```python
from build123d import *

# Parameters (mm, degrees)
F1_DEPTH    = 48
F2_DEPTH    = 10
F3_R        = 6
F4_T1_DEPTH = 30
F5_R        = 6
F6_DEPTH    = 3
F5_W        = 28
F5_H        = 5
F7_DEPTH    = 5
F8_DEPTH    = 25


# Not quite as in the source:
# - a fillet or chamfer that OpenCascade refuses, or shapes differently, is made with other operations: its cross-section is extruded or revolved along the edge and cut away or added


with BuildPart() as f1:
    # F0 (on Front) → F1 (new body)
    with BuildSketch(Plane.XZ):
        Polygon((-21, 43), (-31, 43), (-31, 13), (31, 13), (31, 43), (21, 43), (21, 23), (-21, 23), align=None)
    extrude(amount=F1_DEPTH)

    # F0 (on Front) → F2 (join)
    with BuildSketch(Plane.XZ):
        Polygon((-31, 43), (-46, 43), (-46, 0), (46, 0), (46, 43), (31, 43), (31, 13), (-31, 13), align=None)
        Polygon((-21, 43), (-31, 43), (-31, 13), (31, 13), (31, 43), (21, 43), (21, 23), (-21, 23), align=None)
    extrude(amount=F2_DEPTH)

    # F3
    f3_edges = [f1.edges().sort_by_distance(p)[0] for p in [
        (-46, -5, 0),
        (46, -5, 0),
    ]]
    fillet(f3_edges, radius=F3_R)

    # F4: fillet of radius 25 on 2 edges, made by hand

    # F4_s2 → F4_t1 (join)
    with BuildSketch(Plane.XY.offset(13)):
        with BuildLine():
            ThreePointArc((-46, -10), (-35.0834993366, -19.2198145372), (-31, -32.9128784748))
            Line((-31, -32.9128784748), (-31, -10))
            Line((-31, -10), (-46, -10))
        make_face()
        with BuildLine():
            ThreePointArc((46, -10), (35.0834993366, -19.2198145372), (31, -32.9128784748))
            Line((31, -32.9128784748), (31, -10))
            Line((31, -10), (46, -10))
        make_face()
    extrude(amount=F4_T1_DEPTH)

    # F5 (on face) → F6 (join)
    with BuildSketch(Plane(origin=(0, 0, 13), x_dir=(1, 0, 0), z_dir=(0, 0, -1))):
        with BuildLine():
            Line((14, 15), (14, 29))
            ThreePointArc((14, 29), (0, 43), (-14, 29))
            Line((-14, 29), (-14, 15))
            Line((-14, 15), (14, 15))
        make_face()
        with Locations((0, 29)):
            Circle(F5_R, mode=Mode.SUBTRACT)
    extrude(amount=F6_DEPTH)

    # F5 (on face) → F7 (join)
    with BuildSketch(Plane(origin=(0, 0, 13), x_dir=(1, 0, 0), z_dir=(0, 0, -1))):
        with Locations((0, 12.5)):
            Rectangle(F5_W, F5_H)
    extrude(amount=F7_DEPTH)

    # F5 (on face) → F8 (cut)
    with BuildSketch(Plane(origin=(0, 0, 13), x_dir=(1, 0, 0), z_dir=(0, 0, -1))):
        with Locations((0, 29)):
            Circle(F5_R)
    extrude(amount=-F8_DEPTH, mode=Mode.SUBTRACT)


solid = f1.part
```
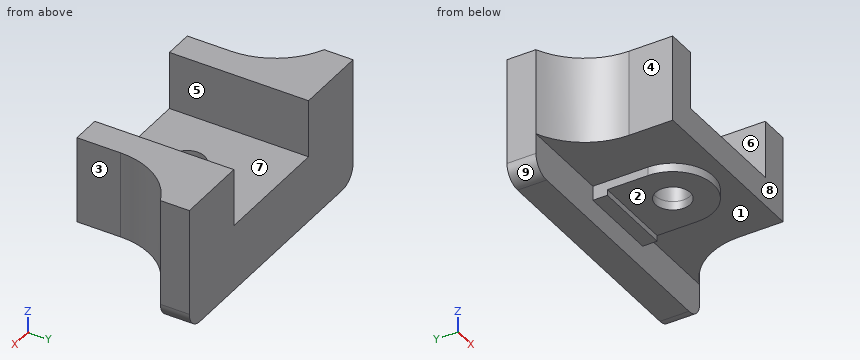
Work out the finished part from the listing and answer in its coordinate system (mm). Face numbers are marked on the shaded views. A direction names the side the tool comes from. Give positions to 0.01 mm unless a question says otherwise; leave off trailing zeros. Loops run counter-clockwise (first coordinate to the right, second up) from the corner with the lowest first, then second, coordinate; pieces in that order, holes last. Notation, with made-up numbers: (16.25, 37) -> (24.25, 37) arc R10 cw to (24.25, 43) -> close; hole circle Ø3 at (-37.75, 19.5). An arc over 180 degrees is marked (long way). Put each result on its own line as item: value. Start each with the question number.
Item 1: The part is cut by section B-B (z = 14). Give the vertices of the cut face in (x, y).
Item 2: Each of these flat-tipped pins is pushed along its axis until it touches: P1, Ø7.5, axis at y = -37.5, z = 29.5, coming from the -X side; P2, Ø4, axis at x = 4.5, y = -13, coming from the -Z side; P3, Ø12, axis at y = -33, z = 29.5, coming from the -X side. Where does it stop, or does it pass through?
Item 3: The part is cut by section D-D (y = -38). Give the vertices of the cut face in (x, z), then the cut area to 3 significant figures.
Item 4: Find the intervals of material crossed by L1, parallel to Y at x = 0, z = 20; L2, parallel to Y at x = 0, z = 10.95; L3, parallel to X at y = -3.5, z = 25, in increasing order. Write a range as [from, to].
Item 5: The mould has two halves that part along X. Classify the marked faces 6, 7, 8 and 9: released by +X, released by -X, zero draft, split by the parting line, or undercut.
Item 6: The part is cut by section C-C (y = -26). Give the vertices of the cut face in (x, z), then the cut area to 3 significant figures.
Item 7: Which of the six approach directions +Z, -Z, +X, -X, +Y, -Y give full straight-line access (tool end or side, diameter ignored) to the marked faces 1, 2, 3, 4 and 5?
Item 8: The part is cut by section A-A (x = 0). Give the vertices of the cut face in (y, z).
Answers below:
1. outline: (-46, -10) arc R25 cw to (-31, -32.91) -> (-31, -48) -> (31, -48) -> (31, -32.91) arc R25 cw to (46, -10) -> (46, 0) -> (-46, 0) -> close; hole circle Ø12 at (0, -29)
2. P1: x = -31
2. P2: z = 8
2. P3: x = -31.71
3. outline: (-31, 13) -> (-10.72, 13) -> (-10.72, 10) -> (10.72, 10) -> (10.72, 13) -> (31, 13) -> (31, 43) -> (21, 43) -> (21, 23) -> (-21, 23) -> (-21, 43) -> (-31, 43) -> close
3. area: 1,080 mm2
4. L1: [-48, -35], [-23, 0]
4. L2: [-43, -35], [-23, 0]
4. L3: [-46, -21], [21, 46]
5. face 6: undercut
5. face 7: undercut
5. face 8: zero draft
5. face 9: released by -X
6. outline: (-31.97, 13) -> (-14, 13) -> (-14, 10) -> (-5.2, 10) -> (-5.2, 23) -> (-21, 23) -> (-21, 43) -> (-31.97, 43) -> close; (5.2, 10) -> (14, 10) -> (14, 13) -> (31.97, 13) -> (31.97, 43) -> (21, 43) -> (21, 23) -> (5.2, 23) -> close
6. area: 1,030 mm2
7. face 1: -Z, -Y
7. face 2: -Z, +X, -X, -Y
7. face 3: +Z, -Z, +X, -Y
7. face 4: +Z, -Z, -X, -Y
7. face 5: +Z, +Y, -Y
8. outline: (-48, 13) -> (-43, 13) -> (-43, 10) -> (-35, 10) -> (-35, 23) -> (-48, 23) -> close; (-23, 10) -> (-15, 10) -> (-15, 8) -> (-10, 8) -> (-10, 0) -> (0, 0) -> (0, 23) -> (-23, 23) -> close
